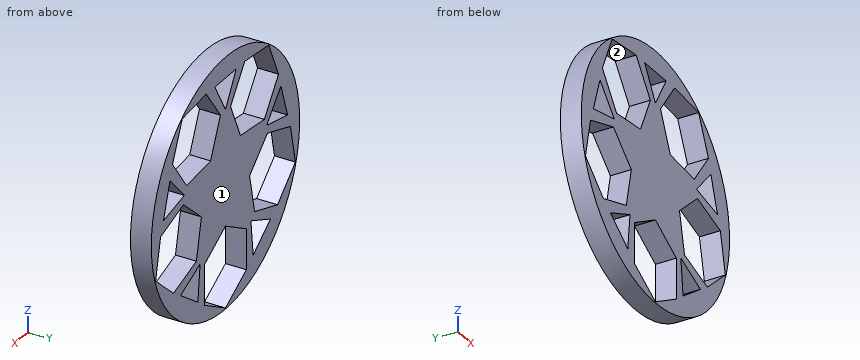
```python
from build123d import *

# Parameters (mm, degrees)
F0_R     = 152.4
F2_DEPTH = 25.4


# Not quite as in the source:
# - a feature of the source that left no trace in its solid (it failed there, or was rolled back) is left out


with BuildPart() as f2:
    # F0 (on Front) → F2 (new body)
    with BuildSketch(Plane.XZ):
        Circle(F0_R)
        Polygon((-52.2541089288, -71.9216107999), (-56.8527436029, -115.6746970812), (-92.4447104794, -89.8156194901), align=None, mode=Mode.SUBTRACT)
        Polygon((-59.8193788497, -64.5381655614), (-106.9252081018, -79.8437772928), (-143.7331713077, -46.7017383599), (-133.4353052615, 1.7459123045), (-86.3294760094, 17.0515240359), (-49.5215128035, -16.0905148971), align=None, mode=Mode.SUBTRACT)
        Polygon((42.8942382494, -76.835), (42.8942382494, -126.365), (0, -151.13), (-42.8942382494, -126.365), (-42.8942382494, -76.835), (0, -52.07), align=None, mode=Mode.SUBTRACT)
        Polygon((52.2541089288, -71.9216107999), (92.4447104794, -89.8156194901), (56.8527436029, -115.6746970812), align=None, mode=Mode.SUBTRACT)
        Polygon((86.3294760094, 17.0515240359), (133.4353052615, 1.7459123045), (143.7331713077, -46.7017383599), (106.9252081018, -79.8437772928), (59.8193788497, -64.5381655614), (49.5215128035, -16.0905148971), align=None, mode=Mode.SUBTRACT)
        Polygon((-84.5489242986, 27.4716107999), (-127.5816383797, 18.3247250555), (-113.9867167593, 60.1655915157), align=None, mode=Mode.SUBTRACT)
        Polygon((-79.8646475645, 36.9482201115), (-108.9776511105, 77.0188318428), (-88.831985179, 122.2667383599), (-39.5733157014, 127.4440331455), (-10.4603121553, 87.3734214141), (-30.6059780869, 42.1255148971), align=None, mode=Mode.SUBTRACT)
        Polygon((84.5489242986, 27.4716107999), (113.9867167593, 60.1655915157), (127.5816383797, 18.3247250555), align=None, mode=Mode.SUBTRACT)
        Polygon((21.9970452561, 127), (0, 88.9), (-21.9970452561, 127), align=None, mode=Mode.SUBTRACT)
        Polygon((10.4603121553, 87.3734214141), (39.5733157014, 127.4440331455), (88.831985179, 122.2667383599), (108.9776511105, 77.0188318428), (79.8646475645, 36.9482201115), (30.6059780869, 42.1255148971), align=None, mode=Mode.SUBTRACT)
    extrude(amount=F2_DEPTH)


solid = f2.part
```
Build history of the part. All positions in model axes, mm. Face numbers are marked on the shaded views. Give positions to 0.01 mm unless a question says otherwise; leave off trailing zeros. Order: outer loops, then holes, each group sorted by start corner. A loop starts at its lowest first (then second) coordinate and runs counter-clockwise, first axis right, second up. Notation, with made-up numbers: M 16.5,19.5 L 69.5,19.5 A12 cw 69.5,29.5 Z; hole C 84,71.25 d2. An arc over 180 degrees is marked long. Return JSON: item names as keys, results as strings.
Q1. Wall check: probe 1 along Z at (x, y) = (40.5, -4.75); probe 2 along X at (y, z) = (-9.5, -18.5); probe 3 along X at (y, z) = (-4.25, 92). Give the ranges that are in metal, low to high. Write a range as from..to.
Answer list:
{"probe 1": "z = -146.92..-127.75, -75.45..41.09, 127.35..146.92", "probe 2": "x = -151.27..-137.74, -50.03..50.03, 137.74..151.27", "probe 3": "x = -121.5..-102.31, -13.82..-1.79, 1.79..13.82, 102.31..121.5"}
Q2. Band-saw the part on A-A (z = 98.5). Give the cut face in (x, y), then the cut area to 3 significant figures.
Answer list:
{"outline": "M -116.29,-25.4 L -99.41,-25.4 L -99.41,0 L -116.29,0 Z; M -18.54,-25.4 L -5.54,-25.4 L -5.54,0 L -18.54,0 Z; M 5.54,-25.4 L 18.54,-25.4 L 18.54,0 L 5.54,0 Z; M 99.41,-25.4 L 116.29,-25.4 L 116.29,0 L 99.41,0 Z", "area": "1,520 mm^2"}
Q3. Band-saw the part on C-C (x = -117.5). Give the cut face in (y, z).
Answer list:
{"outline": "M -25.4,-97.05 L 0,-97.05 L 0,-70.32 L -25.4,-70.32 Z; M -25.4,6.92 L 0,6.92 L 0,20.47 L -25.4,20.47 Z; M -25.4,49.35 L 0,49.35 L 0,97.05 L -25.4,97.05 Z"}
Q4. Flat gauge pins, fed straight in: pin 1 (6 mm diameter, centred on x = -49, y = -10, fed in from -Z); pin 2 (4 mm diameter, centred on y = -8, z = 94.5, fed in from +X); pin 3 (8 mm diameter, centred on y = -5, z = -46.5, fed in from +X); pin 4 (8 mm diameter, centred on x = 63.5, z = 121.5, fed in from -Y). Where does each tip first touch, or does it go through?
Answer list:
{"pin 1": "stops at z = -145.29", "pin 2": "stops at x = 121.12", "pin 3": "stops at x = 146.35", "pin 4": "stops at y = -25.4"}
Q5. Two-plate mould, pull along Z, no slides. Class the marked faces 1 and 2: pulls with the +Z half, pulls with the -Z half, needs draft (parallel to the pull), parting line crosses it, or undercut.
Answer list:
{"face 1": "needs draft", "face 2": "undercut"}
Q6. Band-saw the part on D-D (z = -5.5). Give the cut face in (x, y), then the cut area to 3 significant figures.
Answer list:
{"outline": "M -152.3,-25.4 L -134.98,-25.4 L -134.98,0 L -152.3,0 Z; M -61.28,-25.4 L 61.28,-25.4 L 61.28,0 L -61.28,0 Z; M 134.98,-25.4 L 152.3,-25.4 L 152.3,0 L 134.98,0 Z", "area": "3,990 mm^2"}
Q7. Band-saw the part on B-B (y = -12). Count the separate pieces of the cut face and the enclosed holes in it, then the cut area to 3 significant figures.
Answer list:
{"separate pieces": "1", "enclosed holes": "10", "area": "36,900 mm^2"}
